Here's how the part is built. I have some questions about the finished solid (model axes, mm). A direction names the side the tool comes from. Coordinates: 2 decimals unless noted, no trailing zeros. Write each loop counter-clockwise with the first axis right and the second up, starting at its lowest first coordinate (ties: lowest second). Pieces come first, ordered by that corner, then holes. Notation, with made-up numbers: (12.5, 29) - (68.5, 29) arc R26 ccw to (68.5, 66) - close; hole circle Ø1 at (-14.75, 1). An arc over 180 degrees is marked (long way). Answer in a Markdown table with one row per item. Add a question column.
Item 1: We'd pull the mould along Z, two halves only. Please class faces 3 (the face through (-2, 2, 0)), 4 (the face through (34.5, 69.8, 71.3)), 5 (the face through (104, 70, 30)): +Z half, -Z half, draft (parallel to the pull), parting line (faces both ways), or undercut.
Item 2: If I drill on probe 1 along Y at (x, z) = (130.5, 37.5); probe 2 along Z at (x, y) = (-12, 55.5); probe 3 along Y at (x, z) = (120, 15.5), over which ranges is the centre line in solid material (lowest first)? Write a range as from..to.
Item 3: Which directions (+Z, -Z, +X, -X, +Y, -Y) give clear straight access to the entire face, cutting with the end or side of a thin tool? Please do faces 1 (the face through (104, 100, 8)), 2 (the face through (70, 107.5, 28)).
Item 4: Imagine slicing it at D-D (x = 89). Please give me the cut outline in (y, z), plus the area to 3 significant figures.
Item 5: Imagine slicing it at C-C (z = 21.5). Please give me the cut outline in (x, y), plus the area to 3 significant figures.
Item 6: I'm going to push flat-ended pins straight in: pin 1 (1.5 mm diameter, centred on x = -59, y = 32, fed in from -Z); pin 2 (21 mm diameter, centred on y = 84, z = 28.5, fed in from +X); pin 3 (8 mm diameter, centred on x = 8, y = -79, fed in from +Z); pin 4 (12 mm diameter, centred on x = 80.5, z = 41, fed in from -Y). Where does each tip first touch, or does it pass through?
Item 7: Imagine slicing it at B-B (x = 51). Please give me the cut outline in (y, z), plus the area to 3 significant figures.
Item 8: Imagine slicing it at A-A (y = 83). Please give me the cut outline in (x, z).
from build123d import *
from build123d import SkipClean  # not in build123d's __all__

# Parameters (mm, degrees)
F1_DEPTH = 46
F3_DEPTH = 74
F4_DEPTH = 143.5


with BuildPart() as f1:
    # F0 (on Top) → F1 (new body)
    with BuildSketch(Plane.XY):
        with BuildLine():
            Line((178, 107.5), (0, 107.5))
            ThreePointArc((0, 107.5), (-65.1632565178, -85.4985379992), (103.6532681588, 28.5))
            Line((103.6532681588, 28.5), (178, 28.5))
            Line((178, 28.5), (178, 107.5))
        make_face()
    extrude(amount=F1_DEPTH)

    # F2 (on face) → F3 (cut)
    with BuildSketch(Plane.YZ.offset(178)):
        with BuildLine():
            ThreePointArc((70, 0), (40.6316496888, 14.1815523673), (33.4760352645, 46))
            Line((33.4760352645, 46), (28.5, 46))
            Line((28.5, 46), (28.5, 0))
            Line((28.5, 0), (70, 0))
        make_face()
        with BuildLine():
            Line((107.5, 0), (107.5, 37.5))
            ThreePointArc((107.5, 37.5), (96.5165042945, 10.9834957055), (70, 0))
            Line((70, 0), (107.5, 0))
        make_face()
        with BuildLine():
            ThreePointArc((37.596296508, 46), (65.714796795, 4.275204538), (103.5, 37.5))
            ThreePointArc((103.5, 37.5), (103.224795462, 41.785203205), (102.403703492, 46))
            Line((102.403703492, 46), (37.596296508, 46))
        make_face()
    extrude(amount=-F3_DEPTH, mode=Mode.SUBTRACT)

    # F2 (on face) → F4 (join)
    with BuildSketch(Plane.YZ.offset(178)):
        with BuildLine():
            ThreePointArc((37.596296508, 46), (70, 71), (102.403703492, 46))
            Line((102.403703492, 46), (106.5239647355, 46))
            ThreePointArc((106.5239647355, 46), (70, 75), (33.4760352645, 46))
            Line((33.4760352645, 46), (37.596296508, 46))
        make_face()
    with SkipClean():  # cleaning this boolean's faces spoils the solid; the shape is the same uncleaned
        extrude(amount=-F4_DEPTH)


solid = f1.part
Here are the results:
| question | item | result |
|---|---|---|
| 1 | face 3 | -Z half |
| 1 | face 4 | draft |
| 1 | face 5 | undercut |
| 2 | probe 1 | y = 32.5..36.5, 103.5..107.5 |
| 2 | probe 2 | z = 0..46 |
| 2 | probe 3 | y = 39.63..44.74, 95.26..100.37 |
| 3 | face 1 | -Z, +X, +Y |
| 3 | face 2 | +Z, -Z, +X, -X, +Y |
| 4 | outline | (-60.29, 0) - (107.5, 0) - (107.5, 46) - (106.52, 46) arc R37.5 ccw to (33.48, 46) - (-60.29, 46) - close; hole (37.6, 46) - (102.4, 46) arc R33.5 ccw to start |
| 4 | area | 8,100 mm2 |
| 5 | outline | (0, 107.5) arc R107.5 ccw (long way) to (103.65, 28.5) - (104, 28.5) - (104, 36.08) - (178, 36.08) - (178, 40.57) - (104, 40.57) - (104, 99.43) - (178, 99.43) - (178, 103.92) - (104, 103.92) - (104, 107.5) - close |
| 5 | area | 39,100 mm2 |
| 6 | pin 1 | stops at z = 0 |
| 6 | pin 2 | stops at x = 104 |
| 6 | pin 3 | stops at z = 46 |
| 6 | pin 4 | stops at y = -77.5 |
| 7 | outline | (-94.63, 0) - (107.5, 0) - (107.5, 46) - (106.52, 46) arc R37.5 ccw to (33.48, 46) - (-94.63, 46) - close; hole (37.6, 46) - (102.4, 46) arc R33.5 ccw to start |
| 7 | area | 9,680 mm2 |
| 8 | outline | (-68.32, 0) - (104, 0) - (104, 2.33) - (178, 2.33) - (178, 6.63) - (104, 6.63) - (104, 46) - (-68.32, 46) - close; (34.5, 68.37) - (178, 68.37) - (178, 72.67) - (34.5, 72.67) - close |
